```python
from build123d import *

# Parameters (mm, degrees)
F1_DEPTH = 19.05
F3_DEPTH = 9.525
F5_DEPTH = 28.576
F6_R     = 7.62
F7_DEPTH = 9.525
F9_DEPTH = 9.525


with BuildPart() as f1:
    # F0 (on Top) → F1 (new body)
    with BuildSketch(Plane.XY):
        Polygon((53.975, 9.525), (0, 9.525), (-53.975, 9.525), (-53.975, -9.525), (-9.525, -9.525), (-9.525, -85.725), (0, -85.725), (9.525, -85.725), (9.525, -9.525), (53.975, -9.525), align=None)
    extrude(amount=F1_DEPTH)

    # F2 (on face) → F3 (join)
    with BuildSketch(Plane.XY.offset(19.05)):
        Polygon((47.625, 3.175), (-47.625, 3.175), (-47.625, -3.175), (-3.175, -3.175), (-3.175, -79.375), (3.175, -79.375), (3.175, -3.175), (47.625, -3.175), align=None)
    extrude(amount=F3_DEPTH)

    # F4 (on face) → F5 (cut, through all)
    with BuildSketch(Plane.XY.offset(28.575)):
        with BuildLine():
            ThreePointArc((-3.175, -55.7836379401), (0, -58.9586379401), (3.175, -55.7836379401))
            Line((3.175, -55.7836379401), (3.175, -30.3836379401))
            ThreePointArc((3.175, -30.3836379401), (0, -27.2086379401), (-3.175, -30.3836379401))
            Line((-3.175, -30.3836379401), (-3.175, -55.7836379401))
        make_face()
        with BuildLine():
            ThreePointArc((-19.05, 3.175), (-22.225, 0), (-19.05, -3.175))
            Line((-19.05, -3.175), (0, -3.175))
            Line((0, -3.175), (19.05, -3.175))
            ThreePointArc((19.05, -3.175), (22.225, 0), (19.05, 3.175))
            Line((19.05, 3.175), (0, 3.175))
            Line((0, 3.175), (-19.05, 3.175))
        make_face()
    extrude(amount=-F5_DEPTH, mode=Mode.SUBTRACT)

    # F6 (on face) → F7 (cut)
    with BuildSketch(Plane.XY.offset(28.575)):
        with BuildLine():
            ThreePointArc((-25.9770321928, -3.175), (-17.4251285142, -7.4447426184), (-11.43, 0))
            ThreePointArc((-11.43, 0), (-17.4251285142, 7.4447426184), (-25.9770321928, 3.175))
            Line((-25.9770321928, 3.175), (-19.05, 3.175))
            ThreePointArc((-19.05, 3.175), (-22.225, 0), (-19.05, -3.175))
            Line((-19.05, -3.175), (-25.9770321928, -3.175))
        make_face()
        with Locations((19.05, 0)):
            Circle(F6_R)
        with Locations((0, -30.3836379401)):
            Circle(F6_R)
        with Locations((0, -55.7836379401)):
            Circle(F6_R)
        with BuildLine():
            Line((-19.05, 3.175), (-25.9770321928, 3.175))
            ThreePointArc((-25.9770321928, 3.175), (-26.67, 0), (-25.9770321928, -3.175))
            Line((-25.9770321928, -3.175), (-19.05, -3.175))
            ThreePointArc((-19.05, -3.175), (-22.225, 0), (-19.05, 3.175))
        make_face()
        Circle(F6_R)
    extrude(amount=-F7_DEPTH, mode=Mode.SUBTRACT)

    # F8 (on face) → F9 (cut, through all)
    with BuildSketch(Plane.XY.offset(28.575)):
        with BuildLine():
            Line((-25.9770321928, 3.175), (-47.625, 3.175))
            Line((-47.625, 3.175), (-47.625, -3.175))
            Line((-47.625, -3.175), (-25.9770321928, -3.175))
            ThreePointArc((-25.9770321928, -3.175), (-26.67, 0), (-25.9770321928, 3.175))
        make_face()
        with BuildLine():
            Line((47.625, 3.175), (25.9770321928, 3.175))
            ThreePointArc((25.9770321928, 3.175), (26.67, 0), (25.9770321928, -3.175))
            Line((25.9770321928, -3.175), (47.625, -3.175))
            Line((47.625, -3.175), (47.625, 3.175))
        make_face()
    extrude(amount=-F9_DEPTH, mode=Mode.SUBTRACT)


solid = f1.part
```
CAD build for the part. Positions are in the model's coordinates, mm. A direction names the side the tool comes from. Give positions to 0.01 mm unless a question says otherwise; leave off trailing zeros. Write each loop counter-clockwise with the first axis right and the second up, starting at its lowest first coordinate (ties: lowest second). Pieces come first, ordered by that corner, then holes. Notation, with made-up numbers: (68.25, 30.5) -> (81.25, 30.5) arc R16 cw to (81.25, 48.5) -> close; hole circle Ø4 at (35.25, 13). An arc over 180 degrees is marked (long way). Write each question's results on one line, items separated by ' | '.
1. Which spindle directions (+Z, -Z, +X, -X, +Y, -Y) get a long thin tool onto all of the face, cutting with end or side? Do faces 4 (the flat face through (31, -9.525, 9)), 5 (the flat face through (3.175, -71, 24)), 6 (the cylindrical face through (-0.046, -63.404, 23.879)), 7 (the cylindrical face through (-0.07, -58.958, 9.658)). Say none if no direction does.
Geometry check:
face 4: +Z, -Z, +X, -Y | face 5: +Z, +X, +Y, -Y | face 6: +Z | face 7: +Z, -Z
2. Cut at C-C, the plane x = 0. Write the cut outline in (y, z) (3 decimals).
Geometry check:
outline: (-85.725, 0) -> (-58.959, 0) -> (-58.959, 19.05) -> (-63.404, 19.05) -> (-63.404, 28.575) -> (-79.375, 28.575) -> (-79.375, 19.05) -> (-85.725, 19.05) -> close; (-27.209, 0) -> (-3.175, 0) -> (-3.175, 19.05) -> (-7.62, 19.05) -> (-7.62, 28.575) -> (-22.764, 28.575) -> (-22.764, 19.05) -> (-27.209, 19.05) -> close; (3.175, 0) -> (9.525, 0) -> (9.525, 19.05) -> (3.175, 19.05) -> close
3. Two-plate mould, pull along Y, no slides. Class faces 1 (the cylindrical face through (-22.224, 0.07, 9.658)), 2 (the flat face through (0, -71, 28.575)), 3 (the flat face through (1, 9.525, 9)): pulls with the +Y half, pulls with the -Y half, needs draft (parallel to the pull), parting line crosses it, or undercut.
Geometry check:
face 1: undercut | face 2: needs draft | face 3: pulls with the +Y half
4. Cut at D-D, the plane z = 10.5. Write the cut outline in (x, y) (3 decimals).
Geometry check:
outline: (-53.975, -9.525) -> (-9.525, -9.525) -> (-9.525, -85.725) -> (9.525, -85.725) -> (9.525, -9.525) -> (53.975, -9.525) -> (53.975, 9.525) -> (-53.975, 9.525) -> close; hole (-19.05, -3.175) -> (19.05, -3.175) arc R3.175 ccw to (19.05, 3.175) -> (-19.05, 3.175) arc R3.175 ccw to start; hole (-3.175, -55.784) arc R3.175 ccw to (3.175, -55.784) -> (3.175, -30.384) arc R3.175 ccw to (-3.175, -30.384) -> close
5. Wall check: probe 1 along Y at (x, z) = (-18, 15.25) (3 decimals); probe 2 along Y at (x, z) = (-43.5, 17.75) (3 decimals). Give the ranges that are in metal, low to high. Write a range as [from, to].
Geometry check:
probe 1: [-9.525, -3.175], [3.175, 9.525] | probe 2: [-9.525, 9.525]
6. Drop flat-ended pins along their axis: P1, Ø9.5, axis at y = -31.5, z = 11, coming from the -X side (3 decimals); P2, Ø7.5, axis at y = -15.5, z = 25, coming from the -X side (3 decimals); P3, Ø5.5, axis at y = -38.5, z = 6, coming from the +X side (3 decimals); P4, Ø1.5, axis at y = -10, z = 11.5, coming from the +X side (3 decimals). Give the stop position or say it passes through.
Geometry check:
P1: x = -9.525 | P2: x = -3.175 | P3: x = 9.525 | P4: x = 53.975
7. Cut at A-A, the plane y = -39.5. Write the cut outline in (x, z) (3 decimals), then the cut area to 3 significant figures.
Geometry check:
outline: (-9.525, 0) -> (-3.175, 0) -> (-3.175, 19.05) -> (-9.525, 19.05) -> close; (3.175, 0) -> (9.525, 0) -> (9.525, 19.05) -> (3.175, 19.05) -> close | area: 242 mm²
